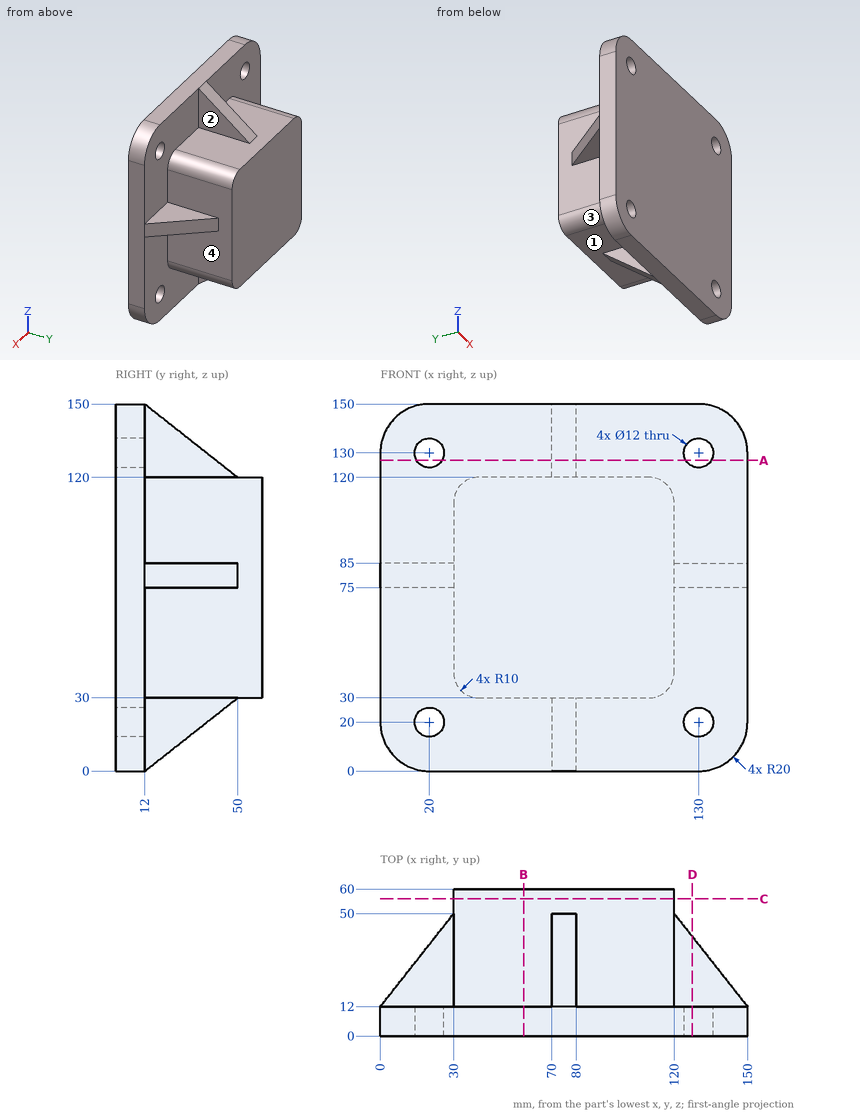
Source: three-view drawing plus pictorial views. Frame: mm from the lowest corner of the part. A direction names the side the tool comes from. Coordinates: 2 decimals unless noted, no trailing zeros. Loops run counter-clockwise (first coordinate to the right, second up) from the corner with the lowest first, then second, coordinate; pieces in that order, holes last. Notation, with made-up numbers: (-2.5, 44.25) -> (25.5, 44.25) arc R24 cw to (25.5, 83.25) -> close; hole circle Ø5 at (87, 2). An arc over 180 degrees is marked (long way). Answer in a Markdown table with one row per item. Add a question column.
Q1. Ray query, line 1 along Z through (x, y) = (130, 9); line 2 along X through (y, z) = (48, 48.5). Return the intervals inside material, ascending.
Q2. Section D-D on x = 127.5. Return the cut outline in (y, z), and give its area (3 significant figures).
Q3. Section A-A on z = 127. Return the cut outline in (x, y), and give its area (3 significant figures).
Q4. Section B-B on x = 58.5. Return the cut outline in (y, z).
Q5. Section C-C on y = 56. Return the cut outline in (x, z).
Q6. Reachability of the marked faces 1, 2, 3 and 4 from +Z, -Z, +X, -X, +Y, -Y: full face, straight path, thin tool, end or side. Return the list, or none.
Q7. Contact query for flat-ended pins moving along their axis: pin 1 Ø1.5 at (x, y) = (37, 15.5) entering from -Z; pin 2 Ø6 at (x, y) = (16.5, 28.5) entering from +Z; pin 3 Ø15 at (x, y) = (142.5, 37) entering from +Z; pin 4 Ø14.5 at (y, z) = (39.5, 86) entering from -X. Output: stop coordinate, or through.
Computed values:
| question | item | result |
|---|---|---|
| 1 | line 1 | z = 0 to 14, 26 to 124, 136 to 150 |
| 1 | line 2 | x = 30 to 120 |
| 2 | outline | (0, 0) -> (12, 0) -> (12, 14.55) -> (0, 14.55) -> close; (0, 25.45) -> (12, 25.45) -> (12, 75) -> (40.5, 75) -> (40.5, 85) -> (12, 85) -> (12, 124.55) -> (0, 124.55) -> close; (0, 135.45) -> (12, 135.45) -> (12, 150) -> (0, 150) -> close |
| 2 | area | 1,820 mm^2 |
| 3 | outline | (0, 0) -> (14.8, 0) -> (14.8, 12) -> (0, 12) -> close; (25.2, 0) -> (124.8, 0) -> (124.8, 12) -> (80, 12) -> (80, 41.13) -> (70, 41.13) -> (70, 12) -> (25.2, 12) -> close; (135.2, 0) -> (150, 0) -> (150, 12) -> (135.2, 12) -> close |
| 3 | area | 1,840 mm^2 |
| 4 | outline | (0, 0) -> (12, 0) -> (12, 30) -> (60, 30) -> (60, 120) -> (12, 120) -> (12, 150) -> (0, 150) -> close |
| 5 | outline | (30, 40) arc R10 ccw to (40, 30) -> (110, 30) arc R10 ccw to (120, 40) -> (120, 110) arc R10 ccw to (110, 120) -> (40, 120) arc R10 ccw to (30, 110) -> close |
| 6 | face 1 | -Z, +Y |
| 6 | face 2 | +Z, +X, +Y |
| 6 | face 3 | -Z, -X, +Y |
| 6 | face 4 | +X, +Y |
| 7 | pin 1 | stops at z = 30.26 |
| 7 | pin 2 | stops at z = 85 |
| 7 | pin 3 | passes through |
| 7 | pin 4 | stops at x = 16.04 |
